CAD build for the part. Positions are in the model's coordinates, mm. A direction names the side the tool comes from. Round coordinates to 2 decimals unless told otherwise and drop trailing zeros. Write each loop counter-clockwise with the first axis right and the second up, starting at its lowest first coordinate (ties: lowest second). Pieces come first, ordered by that corner, then holes. Notation, with made-up numbers: (61.25, -25.5) - (118.25, -25.5) arc R14 cw to (118.25, -13.5) - close; hole circle Ø11 at (16, 36). An arc over 180 degrees is marked (long way). Answer in a Markdown table with one row per item.
Autodesk Inventor part; units mm, degrees
ref_plane "YZ Plane" through (0, 0, 0) normal (1, 0, 0) x (0, 1, 0)
ref_plane "XZ Plane" through (0, 0, 0) normal (0, 1, 0) x (-1, 0, 0)
ref_plane "XY Plane" through (0, 0, 0) normal (0, 0, 1) x (1, 0, 0)
sketch "Sketch1" plane through (0, 0, 0) normal (0, 0, 1) x (1, 0, 0)
  line L0 (12.7, -25.4) -> (-12.7, -25.4)
  line L1 (-12.7, -25.4) -> (-12.7, 25.4)
  line L2 (-12.7, 25.4) -> (12.7, 25.4)
  line L3 (12.7, 25.4) -> (12.7, -25.4)
  line L4 (12.7, -25.4) -> (-12.7, 25.4) construction
  line L5 (-12.7, -25.4) -> (12.7, 25.4) construction
  line L6 (-12.7, 25.4) -> (0, 25.4)
  circle A0 centre (-6.35, -19.05) radius 2.6035
  line L7 (-12.7, 25.4) -> (-3.7, 25.4) construction
  line L8 (-3.7, 25.4) -> (-3.7, -25.4) construction
  line L9 (-3.7, -25.4) -> (-12.7, -25.4) construction
  line L10 (-12.7, -25.4) -> (-12.7, 25.4) construction
  point P0 (0, 0)
  dimension "d0" = 25.4
  dimension "d1" = 50.8
  dimension "d4" = 5.207
  dimension "d5" = 6.35
  dimension "d7" = 9
  dimension "d8" = 6.35
extrude "Extrusion1" add sketch "Sketch1" along normal blind 11.43
sketch "Sketch2" plane through (-12.7, -25.4, 0) normal (-1, 0, 0) x (0, 0, 1)
  line L0 (0, 50.8) -> (0, 0)
  line L1 (0, 0) -> (11.43, 0)
  line L2 (11.43, 50.8) -> (11.43, 0)
  line L3 (0, 50.8) -> (11.43, 50.8)
  line L4 (0, 50.8) -> (11.43, 50.8) construction
  line L5 (5.715, 50.8) -> (5.715, 0) construction
  line L6 (0, 0) -> (11.43, 0) construction
  line L7 (0, 25.4) -> (11.43, 25.4) construction
  line L8 (11.43, 0) -> (11.43, 50.8) construction
  circle A0 centre (5.715, 44.45) radius 2.85
  circle A1 centre (5.715, 29.2354) radius 2.85
  circle A2 centre (5.715, 14.4018) radius 2.85
  dimension "d11" = 5.7
  dimension "d12" = 6.35
  dimension "d13" = 5.7
  dimension "d14" = 15.2146
  dimension "d15" = 5.7
  dimension "d16" = 14.8336
extrude "Extrusion2" cut sketch "Sketch2" against normal blind 9 contours A0 | A1 | A2
sketch "Sketch3" plane through (12.7, -25.4, 0) normal (1, 0, 0) x (0, 0, -1)
  line L0 (0, 0) -> (0, 50.8)
  line L1 (0, 50.8) -> (-11.43, 50.8)
  line L2 (-11.43, 0) -> (-11.43, 50.8)
  line L3 (0, 0) -> (-11.43, 0)
  circle A0 centre (-5.715, 44.45) radius 2.85
  circle A1 centre (-5.715, 29.2354) radius 2.85
  circle A2 centre (-5.715, 14.4018) radius 2.85
  point P0 (0, 25.4)
extrude "Extrusion3" cut sketch "Sketch3" against normal blind 9 contours A0 | A1 | A2
properties part number "Torsion_Spring_Lift"
Q1. Saw through at B-B on x = -7. List the corners of the cut face in (y, z) (3 decimals).
Computed:
| item | result |
|---|---|
| outline | (-25.4, 0) - (-21.571, 0) - (-21.571, 11.43) - (-25.4, 11.43) - close; (-16.529, 0) - (25.4, 0) - (25.4, 11.43) - (-16.529, 11.43) - close; hole circle Ø5.7 at (-10.998, 5.715); hole circle Ø5.7 at (3.835, 5.715); hole circle Ø5.7 at (19.05, 5.715) |
Q2. Flat gauge pins, fed straight in: pin 1 (3 mm diameter, centred on y = 20, z = 6.5, fed in from -X); pin 2 (6.5 mm diameter, centred on y = -11.5, z = 6.5, fed in from +X); pin 3 (4.5 mm diameter, centred on x = -6.35, y = -19.05, fed in from -Z). Where does each tip first touch, or does it go through?
Computed:
| item | result |
|---|---|
| pin 1 | stops at x = -3.7 |
| pin 2 | stops at x = 12.7 |
| pin 3 | passes through |
Q3. Pull direction Z, two halves, no side cores. Call faces 4 (the flat face through (0, 25.4, 6)), 5 (the flat face through (-3.7, -11, 6)), 6 (the flat face through (0, 0, 11.43)): released by +Z, released by -Z, zero draft, split by the parting line, or undercut.
Computed:
| item | result |
|---|---|
| face 4 | zero draft |
| face 5 | undercut |
| face 6 | released by +Z |
Q4. Saw through at D-D on y = 19.05. List the corners of the cut face in (x, z) (3 decimals), then the cut area to 3 significant figures.
Computed:
| item | result |
|---|---|
| outline | (-12.7, 0) - (12.7, 0) - (12.7, 2.865) - (3.7, 2.865) - (3.7, 8.565) - (12.7, 8.565) - (12.7, 11.43) - (-12.7, 11.43) - (-12.7, 8.565) - (-3.7, 8.565) - (-3.7, 2.865) - (-12.7, 2.865) - close |
| area | 188 mm2 |
Q5. 3-axis set-ups, long thin cutter, end or side, ignore diameter. For faces 1 (the cylindrical face through (8.26, 17.32, 7.98)), 2 (the flat face through (-3.7, 4, 6)), 3 (the cylindrical face through (-5.15, -16.74, 5.63)): which of +Z, -Z, +X, -X, +Y, -Y reach the whole face in a straight line?
Computed:
| item | result |
|---|---|
| face 1 | +X |
| face 2 | -X |
| face 3 | +Z, -Z |
Q6. Saw through at A-A on y = -19.05. List the corners of the cut face in (x, z), then the cut area to 3 significant figures.
Computed:
| item | result |
|---|---|
| outline | (-12.7, 0) - (-8.95, 0) - (-8.95, 11.43) - (-12.7, 11.43) - close; (-3.75, 0) - (12.7, 0) - (12.7, 11.43) - (-3.75, 11.43) - close |
| area | 231 mm2 |
Q7. Drill centre lines: line 1 (Y direction, x = 9.25, z = 6); line 2 (Y direction, x = 10.25, z = 3.75); line 3 (Z direction, x = -8.75, y = 20). Where is each one in solid material? Low to high.
Computed:
| item | result |
|---|---|
| line 1 | y = -25.4 to -13.83, -8.16 to 1, 6.67 to 16.21, 21.89 to 25.4 |
| line 2 | y = -25.4 to -13.06, -8.93 to 1.77, 5.9 to 16.99, 21.11 to 25.4 |
| line 3 | z = 0 to 3.03, 8.4 to 11.43 |
